from build123d import *

# Parameters (mm, degrees)
F0_R     = 1.27
F1_DEPTH = 5.08
F2_R     = 0.635
F3_DEPTH = 1.27
F4_R     = 5.07999
F5_R     = 1.2699


# Not quite as in the source:
# - a fillet or chamfer is up to 0.001 mm smaller than in the source, because OpenCascade refuses the exact size


with BuildPart() as f1:
    # F0 (on Right) → F1 (new body)
    with BuildSketch(Plane.YZ):
        with BuildLine():
            ThreePointArc((-2.54, 0), (0, -2.54), (2.54, 0))
            ThreePointArc((2.54, 0), (0, 2.54), (-2.54, 0))
        make_face()
        Circle(F0_R, mode=Mode.SUBTRACT)
        with BuildLine():
            Line((10.16, 0), (2.54, 0))
            ThreePointArc((2.54, 0), (0, -2.54), (-2.54, 0))
            Line((-2.54, 0), (-2.54, -2.54))
            Line((-2.54, -2.54), (-2.54, -5.08))
            Line((-2.54, -5.08), (15.24, -5.08))
            Line((15.24, -5.08), (15.24, 0))
            ThreePointArc((15.24, 0), (12.7, -2.54), (10.16, 0))
        make_face()
        with BuildLine():
            ThreePointArc((15.24, 0), (12.7, 2.54), (10.16, 0))
            ThreePointArc((10.16, 0), (12.7, -2.54), (15.24, 0))
        make_face()
        with Locations((12.7, 0)):
            Circle(F0_R, mode=Mode.SUBTRACT)
        Polygon((-2.54, -5.08), (-2.54, -2.54), (-7.62, -2.54), (-10.16, -2.54), (-10.16, -5.08), align=None)
        Polygon((-10.16, -2.54), (-7.62, -2.54), (-7.62, -1.27), align=None)
    extrude(amount=F1_DEPTH)

    # F2 (on face) → F3 (join)
    with BuildSketch(Plane.XY):
        with Locations((2.54, 6.35)):
            Circle(F2_R)
    extrude(amount=F3_DEPTH)

    # F4 (radius 5.08 in the source; OpenCascade refuses exactly that, so slightly less here)
    f4_edges = [f1.edges().sort_by_distance(p)[0] for p in [
        (2.54, 15.24, -5.08),
    ]]
    fillet(f4_edges, radius=F4_R)

    # F5 (radius 1.27 in the source; OpenCascade refuses exactly that, so slightly less here)
    f5_edges = [f1.edges().sort_by_distance(p)[0] for p in [
        (5.08, 13.752105, -3.592105),
        (0, 13.752105, -3.592105),
        (5.08, 0, 2.54),
        (0, 0, 2.54),
    ]]
    fillet(f5_edges, radius=F5_R)


solid = f1.part
Can you work these out from the model? Positions are in its coordinate system, mm. A direction names the side the tool comes from. Coordinates: 2 decimals unless noted, no trailing zeros. Write each loop counter-clockwise with the first axis right and the second up, starting at its lowest first coordinate (ties: lowest second). Pieces come first, ordered by that corner, then holes. Notation, with made-up numbers: (-13, 71.25) - (6, 71.25) arc R25 ccw to (6, 102.25) - close; hole circle Ø10 at (54, 36). An arc over 180 degrees is marked (long way). Return JSON: item names as keys, results as strings. Group by question number.
Item 1: We'd pull the mould along Z, two halves only. Please class faces 5 (the face through (5.08, 4, -2)), 6 (the face through (2.5, -0.17, 1.26)), 7 (the face through (2.558, 13.712, -3.631)): pulls with the +Z half, pulls with the -Z half, needs draft (parallel to the pull), parting line crosses it, or undercut.
Item 2: If we section it at B-B (x = 3.4): Count the separate pieces of the cut face and the enclosed holes in it, then the cut area to 3 significant figures.
Item 3: Which directions (+Z, -Z, +X, -X, +Y, -Y) give clear straight access to the entire face, cutting with the end or side of a thin tool? Please do faces 1 (the face through (0.362, -2.158, -1.288)), 2 (the face through (3, -2.54, -1)), 3 (the face through (2.46, 6.98, 0.63)), 4 (the face through (4.698, -2.178, -1.288)).
Item 4: I'm going to push flat-ended pins straight in: pin 1 Ø0.8 at (x, z) = (2.5, -1.5) entering from -Y; pin 2 Ø1.4 at (x, y) = (2.5, 6.5) entering from +Z; pin 3 Ø2.5 at (x, y) = (3, -3.5) entering from +Z; pin 4 Ø3.5 at (y, z) = (0, 0) entering from -X. Where does each tip first touch, or does it pass through?
Item 5: Please list where these lines run through material, in increasing order: probe 1 along Z at (x, y) = (2.7, 0); probe 2 along Y at (x, z) = (4.65, 1); probe 3 along Y at (x, z) = (0.9, -0.5).
Item 6: If we section it at C-C (y = 6.35): Write out the boundary of the cut face in (x, z) (3 decimals), then the cut area to 3 significant figures.
Return value:
{
 "1": {"face 5": "needs draft", "face 6": "undercut", "face 7": "pulls with the -Z half"},
 "2": {"separate pieces": "1", "enclosed holes": "2", "area": "116 mm^2"},
 "3": {"face 1": "+Z, -X", "face 2": "+Z, +X, -X", "face 3": "+Z", "face 4": "+Z, +X"},
 "4": {"pin 1": "stops at y = -8.88", "pin 2": "stops at z = 1.27", "pin 3": "stops at z = 1.18", "pin 4": "stops at x = 0"},
 "5": {"probe 1": "z = -5.08 to -1.27, 1.27 to 2.54", "probe 2": "y = -1.98 to -0.78, 0.78 to 1.98, 10.72 to 11.92, 13.48 to 14.68", "probe 3": "y = -2.48 to -1.17, 1.17 to 11.53, 13.87 to 15.16"},
 "6": {"outline": "(0, -3.81) arc R1.27 ccw to (1.27, -5.08) - (3.81, -5.08) arc R1.27 ccw to (5.08, -3.81) - (5.08, 0) - (3.175, 0) - (3.175, 1.27) - (1.905, 1.27) - (1.905, 0) - (0, 0) - close", "area": "26.7 mm^2"}
}
